from build123d import *

# Parameters (mm, degrees)
SKETCH1_W           = 80
SKETCH1_H           = 75
BOSS_EXTRUDE1_DEPTH = 2.3
SKETCH2_W           = 2.3
SKETCH2_H           = 10
CUT_EXTRUDE1_DEPTH  = 10
SKETCH3_R           = 1
CUT_EXTRUDE2_DEPTH  = 10
CUT_EXTRUDE3_DEPTH  = 10
FILLET1_R           = 2


with BuildPart() as part:
    # Sketch1 → Boss-Extrude1 (new body)
    with BuildSketch(Plane(origin=(0, 0, 0), x_dir=(1, 0, 0), z_dir=(0, 1, 0))):
        with Locations((40, 37.5)):
            Rectangle(SKETCH1_W, SKETCH1_H)
    extrude(amount=BOSS_EXTRUDE1_DEPTH)

    # Sketch2 → Cut-Extrude1 (cut)
    with BuildSketch(Plane.XZ):
        with Locations((3.85, -52.5)):
            Rectangle(SKETCH2_W, SKETCH2_H)
        with Locations((3.85, -22.5)):
            Rectangle(SKETCH2_W, SKETCH2_H)
        with Locations((76.15, -52.5)):
            Rectangle(SKETCH2_W, SKETCH2_H)
        with Locations((76.15, -22.5)):
            Rectangle(SKETCH2_W, SKETCH2_H)
    extrude(amount=-CUT_EXTRUDE1_DEPTH, mode=Mode.SUBTRACT)

    # Sketch3 → Cut-Extrude2 (cut)
    with BuildSketch(Plane(origin=(0, 2.3, 0), x_dir=(1, 0, 0), z_dir=(0, 1, 0))):
        with Locations((31.2, 71.1)):
            Circle(SKETCH3_R)
        with Locations((59.1, 71.1)):
            Circle(SKETCH3_R)
        with Locations((15.8, 20.3)):
            Circle(SKETCH3_R)
        with Locations((64.2, 19)):
            Circle(SKETCH3_R)
    extrude(amount=-CUT_EXTRUDE2_DEPTH, mode=Mode.SUBTRACT)

    # Sketch4 → Cut-Extrude3 (cut)
    with BuildSketch(Plane(origin=(0, 2.3, 0), x_dir=(1, 0, 0), z_dir=(0, 1, 0))):
        Polygon((40, 10), (20, 10), (20, 65), (60, 65), (60, 10), align=None)
    extrude(amount=-CUT_EXTRUDE3_DEPTH, mode=Mode.SUBTRACT)

    # Fillet1
    fillet1_edges = [part.edges().sort_by_distance(p)[0] for p in [
        (60, 1.15, -10),
        (20, 1.15, -10),
        (20, 1.15, -65),
        (60, 1.15, -65),
    ]]
    fillet(fillet1_edges, radius=FILLET1_R)


solid = part.part
Work out the finished part from the listing and answer in its coordinate system (mm). A direction names the side the tool comes from. Give positions to 0.01 mm unless a question says otherwise; leave off trailing zeros. Write each loop counter-clockwise with the first axis right and the second up, starting at its lowest first coordinate (ties: lowest second). Pieces come first, ordered by that corner, then holes.
Q1. The part is cut by section C-C on y = 1. State how many separate pieces and enclosed holes the cut face has, and give its area (3 significant figures).
Answer:
separate pieces: 1
enclosed holes: 9
area: 3,700 mm2
Q2. Straight lines are drawn through the part: L1, parallel to X at y = 1.8, z = -71.1; L2, parallel to X at y = 1.85, z = -54; L3, parallel to X at y = 0.55, z = -43. For each, find the intervals that lie inside material, in ascending order.
Answer:
L1: x = 0 to 30.2, 32.2 to 58.1, 60.1 to 80
L2: x = 0 to 2.7, 5 to 20, 60 to 75, 77.3 to 80
L3: x = 0 to 20, 60 to 80
Q3. Given pin 1 (8 mm diameter, centred on x = 22.5, z = -51.5, fed in from -Y); pin 2 (1.2 mm diameter, centred on x = 64.2, z = -19, fed in from -Y), each flat-ended and moving along its own axis, determine where each tip first touches the part or whether it passes through.
Answer:
pin 1: stops at y = 0
pin 2: passes through
Q4. For a pull along Z with two mould halves and no side action, classify faces 1 (the face through (0, 1, -37)), 2 (the face through (77.3, 1, -53)), 3 (the face through (39, 1, -75)) as released by +Z, released by -Z, zero draft, split by the parting line, or undercut.
Answer:
face 1: zero draft
face 2: undercut
face 3: released by -Z
Q5. The part is cut by section D-D on x = 44.5. Give the vertices of the cut face in (y, z).
Answer:
outline: (0, -75) - (2.3, -75) - (2.3, -65) - (0, -65) - close; (0, -10) - (2.3, -10) - (2.3, 0) - (0, 0) - close
Q6. A tool of negligible diameter and unlimited length cuts with its end or side. For faces 4 (the face through (5, 1, -23)), 5 (the face through (66, 2.3, -38)), from which of +Z, -Z, +X, -X, +Y, -Y can it reach the whole face along a straight path? Write none if from no direction.
Answer:
face 4: +Y, -Y
face 5: +Z, -Z, +X, -X, +Y
Q7. The part is cut by section A-A on x = 31.2. Give the vertices of the cut face in (y, z).
Answer:
outline: (0, -75) - (2.3, -75) - (2.3, -72.1) - (0, -72.1) - close; (0, -70.1) - (2.3, -70.1) - (2.3, -65) - (0, -65) - close; (0, -10) - (2.3, -10) - (2.3, 0) - (0, 0) - close
Q8. The part is cut by section B-B on z = -30. Give the vertices of the cut face in (x, y).
Answer:
outline: (0, 0) - (20, 0) - (20, 2.3) - (0, 2.3) - close; (60, 0) - (80, 0) - (80, 2.3) - (60, 2.3) - close
